from build123d import *

# Parameters (mm, degrees)
F0_R     = 2.2225
F0_R_2   = 1.1303
F1_DEPTH = 1.27
F2_R     = 5.715
F2_R_2   = 2.2225
F2_R_3   = 1.1303
F3_DEPTH = 2.54
F4_R     = 2.53999


# Not quite as in the source:
# - a fillet or chamfer is up to 0.001 mm smaller than in the source, because OpenCascade refuses the exact size
# - a feature of the source that left no trace in its solid (it failed there, or was rolled back) is left out


with BuildPart() as f1:
    # F0 (on Front) → F1 (new body)
    with BuildSketch(Plane.XZ):
        Circle(F0_R)
        Circle(F0_R_2, mode=Mode.SUBTRACT)
    extrude(amount=F1_DEPTH)

    # F2 (on face) → F3 (join)
    with BuildSketch(Plane.XZ.offset(1.27)):
        Circle(F2_R)
        Circle(F2_R_2, mode=Mode.SUBTRACT)
        Circle(F2_R_2)
        Circle(F2_R_3, mode=Mode.SUBTRACT)
    extrude(amount=F3_DEPTH)

    # F4 (radius 2.54 in the source; OpenCascade refuses exactly that, so slightly less here)
    f4_edges = [f1.edges().sort_by_distance(p)[0] for p in [
        (-5.715, -3.81, 0),
    ]]
    fillet(f4_edges, radius=F4_R)


solid = f1.part
The listing builds one solid part. Answer for the finished solid, in the listing's coordinates (mm). Round coordinates to 2 decimals unless told otherwise and drop trailing zeros. Order: outer loops, then holes, each group sorted by start corner. A loop starts at its lowest first (then second) coordinate and runs counter-clockwise, first axis right, second up. Notation, with made-up numbers: (-31, 5) -> (-6, 5) arc R12 cw to (-6, 19) -> close; hole circle Ø10 at (21, 83). An arc over 180 degrees is marked (long way). Write each question's results on one line, items separated by ' | '. Start each with the question number.
Q1. Find section D-D (y = -1.8). Determine the outline of the cut face in (x, z), then the cut area to 3 significant figures.
Q2. The mould has two halves that part along Z. Classify faces 1 (the cylindrical face through (-0.245, -1.878, -1.103)), 2 (the cylindrical face through (-0.48, -0.63, -2.17)), 3 (the flat face through (-0.1, -1.27, -2.5)): pulls with the +Z half, pulls with the -Z half, needs draft (parallel to the pull), parting line crosses it, or undercut.
Q3. Straight lines are drawn through the part: probe 1 along Y at (x, z) = (-0.75, -2.75); probe 2 along Z at (x, y) = (0, -2.45); probe 3 along Z at (x, y) = (1, -2.5). For each, find the intervals that lie inside material, in ascending order. Write a range as from..to.
Q4. Each of these flat-tipped pins is pushed along its axis until it touches: pin 1 (2 mm diameter, centred on x = -3.5, z = 1.5, fed in from -Y); pin 2 (1.5 mm diameter, centred on x = -1, y = -2.5, fed in from +Z). Where does it stop, or does it pass through?
Q5. Find section C-C (y = -3.2). Determine the outline of the cut face in (x, z).
Worked answers:
1) outline: circle Ø11.32 at (0, 0); hole circle Ø2.26 at (0, 0) | area: 96.6 mm2
2) face 1: undercut | face 2: parting line crosses it | face 3: needs draft
3) probe 1: y = -3.81..-1.27 | probe 2: z = -5.42..-1.13, 1.13..5.42 | probe 3: z = -5.3..-0.53, 0.53..5.3
4) pin 1: stops at y = -3.81 | pin 2: stops at z = 5.61
5) outline: circle Ø9.65 at (0, 0); hole circle Ø2.26 at (0, 0)
